Read the model definition and answer for the solid it produces. Units are mm, in the model's axes. Face numbers are marked on the shaded views. A direction names the side the tool comes from. Coordinates: 2 decimals unless noted, no trailing zeros. Write each loop counter-clockwise with the first axis right and the second up, starting at its lowest first coordinate (ties: lowest second). Pieces come first, ordered by that corner, then holes. Notation, with made-up numbers: M 26,87.25 L 31,87.25 A26 cw 31,120.25 Z; hole C -10,52.25 d9. An arc over 180 degrees is marked long. Use a Markdown table: item, result. Add a question column.
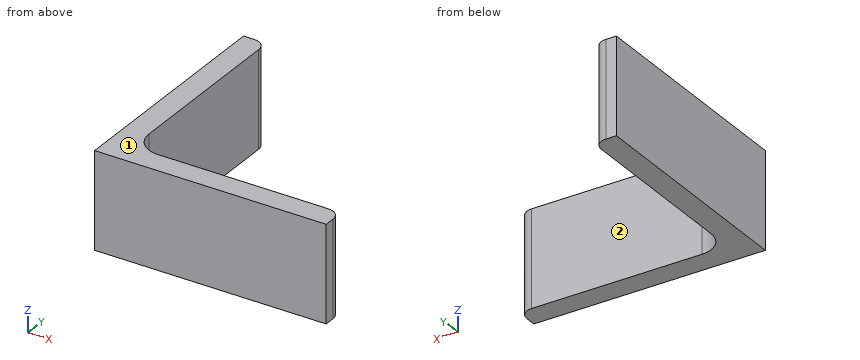
from build123d import *

# Parameters (mm, degrees)
EXTRUDE_DEPTH = 50


with BuildPart() as part:
    # Sketch → Extrude (new body)
    with BuildSketch(Plane.XY):
        with BuildLine():
            Line((0, 0), (120, 0))
            Line((120, 0), (120, 5.5))
            ThreePointArc((120, 5.5), (118.096194, 10.096194), (113.5, 12))
            Line((113.5, 12), (25, 12))
            ThreePointArc((12, 25), (15.807612, 15.807612), (25, 12))
            Line((12, 113.5), (12, 25))
            ThreePointArc((12, 113.5), (10.096194, 118.096194), (5.5, 120))
            Line((0, 120), (5.5, 120))
            Line((0, 0), (0, 120))
        make_face()
    extrude(amount=EXTRUDE_DEPTH)


solid = part.part
Item 1: Each of these flat-tipped pins is pushed along its axis until it touches: pin 1 (10 mm diameter, centred on y = 22, z = 8, fed in from +X); pin 2 (5 mm diameter, centred on y = 108, z = 33, fed in from -X); pin 3 (12 mm diameter, centred on x = 80, z = 21, fed in from +Y). Where does it stop, or does it pass through?
Item 2: Consider probe 1 along X at (y, z) = (39, 41.5); probe 2 along X at (y, z) = (6, 40). Determine where each line is inside the solid, lowest interval first.
Item 3: Find section A-A on z = 8.5. Give the vertices of the cut face in (x, y), then the cut area to 3 significant figures.
Item 4: For the marked faces 1 and 2, determine the directions among +Z, -Z, +X, -X, +Y, -Y from which every point of the face is accessible in a straight line to the end or side of a thin tool.
Item 5: Find section B-B on x = 50.5. Give the vertices of the cut face in (y, z).
Geometry says:
| question | item | result |
|---|---|---|
| 1 | pin 1 | stops at x = 14.75 |
| 1 | pin 2 | stops at x = 0 |
| 1 | pin 3 | stops at y = 12 |
| 2 | probe 1 | x = 0 to 12 |
| 2 | probe 2 | x = 0 to 119.98 |
| 3 | outline | M 0,0 L 120,0 L 120,5.5 A6.5 ccw 113.5,12 L 25,12 A13 cw 12,25 L 12,113.5 A6.5 ccw 5.5,120 L 0,120 Z |
| 3 | area | 2,750 mm2 |
| 4 | face 1 | +Z, +X, -X, +Y, -Y |
| 4 | face 2 | +Z, -Z, +X, +Y |
| 5 | outline | M 0,0 L 12,0 L 12,50 L 0,50 Z |
